Model file for the job. Use its own axes, mm. Face numbers are marked on the shaded views. A direction names the side the tool comes from. Coordinates: 2 decimals unless noted, no trailing zeros. Write each loop counter-clockwise with the first axis right and the second up, starting at its lowest first coordinate (ties: lowest second). Pieces come first, ordered by that corner, then holes. Notation, with made-up numbers: (-14.5, 71.5) -> (23.5, 71.5) arc R35 ccw to (23.5, 103.5) -> close; hole circle Ø3 at (78.5, 67.25). An arc over 180 degrees is marked (long way). Write item = value, one per line. Start each with the question number.
from build123d import *

# Parameters (mm, degrees)
SKETCH_W        = 24.5
SKETCH_H        = 24.5
SKETCH_R        = 1.5
PAD_DEPTH       = 5
SKETCH001_R     = 7.5
PAD001_DEPTH    = 19
SKETCH002_R     = 4
POCKET_DEPTH    = 24.001
CHAMFER_SIZE    = 3
CHAMFER001_SIZE = 3
FILLET_R        = 1
FILLET001_R     = 1
FILLET002_R     = 1


with BuildPart() as part:
    # Sketch → Pad (new body)
    with BuildSketch(Plane.XY):
        Rectangle(SKETCH_W, SKETCH_H)
        with Locations((-8.5, 8.5)):
            Circle(SKETCH_R, mode=Mode.SUBTRACT)
        with Locations((8.5, 8.5)):
            Circle(SKETCH_R, mode=Mode.SUBTRACT)
        with Locations((8.5, -8.5)):
            Circle(SKETCH_R, mode=Mode.SUBTRACT)
        with Locations((-8.5, -8.5)):
            Circle(SKETCH_R, mode=Mode.SUBTRACT)
    extrude(amount=PAD_DEPTH)

    # Sketch001 (on Face10 of Pad) → Pad001 (join)
    with BuildSketch(Plane.XY.offset(5)):
        Circle(SKETCH001_R)
    extrude(amount=PAD001_DEPTH)

    # Sketch002 (on Face12 of Pad001) → Pocket (cut, through all)
    with BuildSketch(Plane.XY.offset(24)):
        Circle(SKETCH002_R)
    extrude(amount=-POCKET_DEPTH, mode=Mode.SUBTRACT)

    # Chamfer
    chamfer_edges = [part.edges().sort_by_distance(p)[0] for p in [
        (12.25, -12.25, 2.5),
        (12.25, 12.25, 2.5),
        (-12.25, 12.25, 2.5),
    ]]
    chamfer(chamfer_edges, length=CHAMFER_SIZE)

    # Chamfer001
    chamfer001_edges = [part.edges().sort_by_distance(p)[0] for p in [
        (-12.25, -12.25, 2.5),
    ]]
    chamfer(chamfer001_edges, length=CHAMFER001_SIZE)

    # Fillet
    fillet_edges = [part.edges().sort_by_distance(p)[0] for p in [
        (-7.5, 0, 24),
    ]]
    fillet(fillet_edges, radius=FILLET_R)

    # Fillet001
    fillet001_edges = [part.edges().sort_by_distance(p)[0] for p in [
        (-4, 0, 24),
    ]]
    fillet(fillet001_edges, radius=FILLET001_R)

    # Fillet002
    fillet002_edges = [part.edges().sort_by_distance(p)[0] for p in [
        (-4, 0, 0),
    ]]
    fillet(fillet002_edges, radius=FILLET002_R)


solid = part.part
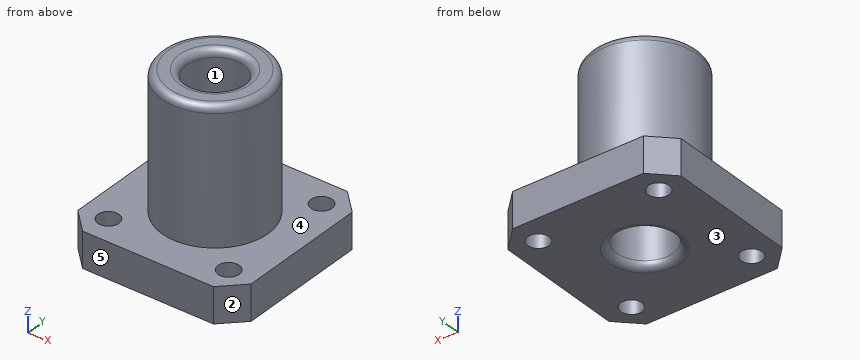
(1) Saw through at D-D (z = 16.5). Give the cut face in (x, y).
(2) 3-axis set-ups, long thin cutter, end or side, ignore diameter. For the marked faces 4 and 5: which of +Z, -Z, +X, -X, +Y, -Y reach the whole face in a straight line?
(3) Drop flat-ended pins along their axis: pin 1 Ø3 at (x, z) = (1, 8) entering from -Y; pin 2 Ø8 at (x, z) = (7, 6.5) entering from +Y; pin 3 Ø12 at (y, z) = (-1.5, 17) entering from +X; pin 4 Ø3.5 at (x, y) = (8.5, -8.5) entering from +Z. Give the stop position or say it passes through.
(4) Mould opens along Y. For the marked faces 1, 2 and 3 say: released by +Y, released by -Y, zero draft, split by the parting line, or undercut.
(5) Drill centre lines: line 1 along Y through (x, z) = (8.5, 2); line 2 along Y through (x, z) = (0, 18.5); line 3 along Z through (x, y) = (5, 6.75). Where is each one in solid material? Low to high.
(6) Saw through at C-C (x = 0). Give the cut face in (y, z), then the cut area to 3 significant figures.
(7) Saw through at A-A (x = 8.5). Give the cut face in (y, z), then the cut area to 3 significant figures.
Returned:
q1.outline = circle Ø15 at (0, 0); hole circle Ø8 at (0, 0)
q2.face_4 = +Z
q2.face_5 = +Z, -Z, +X, -X, -Y
q3.pin_1 = -7.5
q3.pin_2 = 12.25
q3.pin_3 = 7.5
q3.pin_4 = 5
q4.face_1 = undercut
q4.face_2 = released by -Y
q4.face_3 = zero draft
q5.line_1 = -12.25 to -10, -7 to 7, 10 to 12.25
q5.line_2 = -7.5 to -4, 4 to 7.5
q5.line_3 = 0 to 5
q6.outline = (-12.25, 0) -> (-5, 0) arc R1 ccw to (-4, 1) -> (-4, 23) arc R1 ccw to (-5, 24) -> (-6.5, 24) arc R1 ccw to (-7.5, 23) -> (-7.5, 5) -> (-12.25, 5) -> close; (4, 1) arc R1 ccw to (5, 0) -> (12.25, 0) -> (12.25, 5) -> (7.5, 5) -> (7.5, 23) arc R1 ccw to (6.5, 24) -> (5, 24) arc R1 ccw to (4, 23) -> close
q6.area = 214 mm2
q7.outline = (-12.25, 0) -> (-10, 0) -> (-10, 5) -> (-12.25, 5) -> close; (-7, 0) -> (7, 0) -> (7, 5) -> (-7, 5) -> close; (10, 0) -> (12.25, 0) -> (12.25, 5) -> (10, 5) -> close
q7.area = 92.5 mm2
